```python
from build123d import *

# Parameters (mm, degrees)
BOSS_EXTRUDE1_DEPTH = 23
SKETCH2_R           = 18.51
CUT_EXTRUDE1_DEPTH  = 24
SKETCH3_R           = 13.985
CUT_EXTRUDE2_DEPTH  = 7
BOSS_EXTRUDE2_DEPTH = 23
CUT_EXTRUDE3_DEPTH  = 83.130091318
SKETCH10_R          = 3.5
CUT_EXTRUDE5_DEPTH  = 42
CUT_EXTRUDE8_DEPTH  = 83.130091318
CUT_EXTRUDE9_DEPTH  = 9
SKETCH15_R          = 3.5
CUT_EXTRUDE10_DEPTH = 82.477158286


with BuildPart() as part:
    # Sketch1 → Boss-Extrude1 (new body)
    with BuildSketch(Plane(origin=(0, 0, 0), x_dir=(1, 0, 0), z_dir=(0, 1, 0))):
        with BuildLine():
            Line((-100.336081003, -13.275177251), (-7.836081003, 21.091368721))
            ThreePointArc((-7.836081003, 21.091368721), (0, 22.5), (7.836081003, 21.091368721))
            Line((7.836081003, 21.091368721), (100.336081003, -13.275177251))
            ThreePointArc((100.336081003, -13.275177251), (113.745786388, -41.773742524), (85.524728129, -55.758029845))
            Line((85.524728129, -55.758029845), (56.196116933, -46.194642944))
            Line((56.196116933, -46.194642944), (-56.196116933, -46.194642944))
            Line((-56.196116933, -46.194642944), (-85.524728129, -55.758029845))
            ThreePointArc((-85.524728129, -55.758029845), (-113.745786388, -41.773742524), (-100.336081003, -13.275177251))
        make_face()
    extrude(amount=BOSS_EXTRUDE1_DEPTH)

    # Sketch2 → Cut-Extrude1 (cut, through all)
    with BuildSketch(Plane(origin=(0, 23, 0), x_dir=(1, 0, 0), z_dir=(0, 1, 0))):
        with Locations((-92.5, -34.366545972)):
            Circle(SKETCH2_R)
        with Locations((92.5, -34.366545972)):
            Circle(SKETCH2_R)
    extrude(amount=-CUT_EXTRUDE1_DEPTH, mode=Mode.SUBTRACT)

    # Sketch3 → Cut-Extrude2 (cut)
    with BuildSketch(Plane(origin=(0, 23, 0), x_dir=(1, 0, 0), z_dir=(0, 1, 0))):
        Circle(SKETCH3_R)
    extrude(amount=-CUT_EXTRUDE2_DEPTH, mode=Mode.SUBTRACT)

    # Sketch4 → Boss-Extrude2 (add)
    with BuildSketch(Plane(origin=(0, 23, 0), x_dir=(1, 0, 0), z_dir=(0, 1, 0))):
        with BuildLine():
            Line((-113.444632068, -26.146303424), (-132.192515375, -33.11170876))
            Line((-132.192515375, -33.11170876), (-121.744407372, -61.233533721))
            Line((-121.744407372, -61.233533721), (-102.996524064, -54.268128385))
            ThreePointArc((-102.996524064, -54.268128385), (-113.591368721, -42.202626974), (-113.444632068, -26.146303424))
        make_face()
        with BuildLine():
            Line((113.444632068, -26.146303424), (132.192515375, -33.11170876))
            Line((132.192515375, -33.11170876), (121.744407372, -61.233533721))
            Line((121.744407372, -61.233533721), (102.996524064, -54.268128385))
            ThreePointArc((102.996524064, -54.268128385), (113.591368721, -42.202626974), (113.444632068, -26.146303424))
        make_face()
    extrude(amount=-BOSS_EXTRUDE2_DEPTH)

    # Sketch5 → Cut-Extrude3 (cut, through all)
    with BuildSketch(Plane(origin=(5.224054002, 0, 14.060912481), x_dir=(0.937394165, 0, -0.348270267), z_dir=(0.348270267, 0, 0.937394165))):
        with BuildLine():
            Line((-135.448316262, 0), (-135.448316262, 14))
            Line((-135.448316262, 14), (-126.448316262, 14))
            ThreePointArc((-126.448316262, 14), (-133.448316262, 7), (-126.448316262, 0))
            Line((-126.448316262, 0), (-135.448316262, 0))
        make_face()
    extrude(amount=-CUT_EXTRUDE3_DEPTH, mode=Mode.SUBTRACT)

    # Sketch10 → Cut-Extrude5 (cut)
    with BuildSketch(Plane(origin=(5.224054002, 0, 14.060912481), x_dir=(0.937394165, 0, -0.348270267), z_dir=(0.348270267, 0, 0.937394165))):
        with Locations((-126.448316262, 7)):
            Circle(SKETCH10_R)
    extrude(amount=-CUT_EXTRUDE5_DEPTH, mode=Mode.SUBTRACT)

    # Sketch13 → Cut-Extrude8 (cut, through all)
    with BuildSketch(Plane(origin=(-5.224054002, 0, 14.060912481), x_dir=(0.937394165, 0, 0.348270267), z_dir=(-0.348270267, 0, 0.937394165))):
        with BuildLine():
            Line((126.448316262, 14), (135.448316262, 14))
            Line((135.448316262, 14), (135.448316262, 0))
            Line((135.448316262, 0), (126.448316262, 0))
            ThreePointArc((126.448316262, 0), (133.448316262, 7), (126.448316262, 14))
        make_face()
    extrude(amount=-CUT_EXTRUDE8_DEPTH, mode=Mode.SUBTRACT)

    # Sketch14 → Cut-Extrude9 (cut)
    with BuildSketch(Plane(origin=(0, 23, 0), x_dir=(1, 0, 0), z_dir=(0, 1, 0))):
        Polygon((-56.196116933, -46.194642944), (-93.033770242, 18.702535116), (-179.483612129, -24.236128073), (-123.538544412, -84.420295749), align=None)
        Polygon((179.483612129, -24.236128073), (123.538544412, -84.420295749), (56.196116933, -46.194642944), (93.033770242, 18.702535116), align=None)
    extrude(amount=-CUT_EXTRUDE9_DEPTH, mode=Mode.SUBTRACT)

    # Sketch15 → Cut-Extrude10 (cut, through all)
    with BuildSketch(Plane(origin=(-5.224054002, 0, 14.060912481), x_dir=(0.937394165, 0, 0.348270267), z_dir=(-0.348270267, 0, 0.937394165))):
        with Locations((126.448316262, 7)):
            Circle(SKETCH15_R)
    extrude(amount=-CUT_EXTRUDE10_DEPTH, mode=Mode.SUBTRACT)


solid = part.part
```
Read the model definition and answer for the solid it produces. Units are mm, in the model's axes. A direction names the side the tool comes from. Coordinates: 2 decimals unless noted, no trailing zeros. Loops run counter-clockwise (first coordinate to the right, second up) from the corner with the lowest first, then second, coordinate; pieces in that order, holes last. Notation, with made-up numbers: (-28.75, 4.5) - (-6.75, 4.5) arc R15 cw to (-6.75, 22.5) - close; hole circle Ø5 at (0, 40.25). An arc over 180 degrees is marked (long way). Answer in a Markdown table with one row per item.
1. Straight lines are drawn through the part: line 1 (X direction, y = 3.25, z = 26); line 2 (X direction, y = 6.5, z = 33); line 3 (Y direction, x = -74, z = 44). For each, find the intervals that lie inside material, in ascending order.
Conclusion:
| item | result |
|---|---|
| line 1 | x = -113.39 to -109.01, -75.99 to 75.99, 109.01 to 113.39 |
| line 2 | x = -130.08 to -126.33, -118.94 to -110.96, -74.04 to 74.04, 110.96 to 118.94, 126.33 to 130.08 |
| line 3 | y = 0 to 14 |
2. Find section C-C, the plane x = 0. Write down the section's boundary in (y, z) (3 decimals), then the cut area to 3 significant figures.
Conclusion:
| item | result |
|---|---|
| outline | (0, -22.5) - (23, -22.5) - (23, -13.985) - (16, -13.985) - (16, 13.985) - (23, 13.985) - (23, 46.195) - (0, 46.195) - close |
| area | 1,380 mm² |
3. Given pin 1 (6 mm diameter, centred on x = -99, y = 3.5, fed in from -Z); pin 2 (4 mm diameter, centred on y = 10.5, z = 15.5, fed in from -X); pin 3 (8 mm diameter, centred on x = -98.5, y = 11.5, fed in from +Z), each flat-ended and moving along its own axis, determine where each tip first touches the part or whether it passes through.
Conclusion:
| item | result |
|---|---|
| pin 1 | stops at z = 11.66 |
| pin 2 | stops at x = -107.39 |
| pin 3 | stops at z = 56.78 |
4. Find section D-D, the plane x = -106. Write down the section's boundary in (y, z).
Conclusion:
| item | result |
|---|---|
| outline | (0, 16.37) - (14, 16.37) - (14, 21.7) - (0, 21.7) - close; (0, 47.03) - (14, 47.03) - (14, 55.38) - (0, 55.38) - close |
5. Which of the six approach directions +Z, -Z, +X, -X, +Y, -Y give full straight-line access (tool end or side, diameter ignored) to faces 4 (the face through (71.066, 6.902, 51.043)), 5 (the face through (13.34, 19.55, -4.2)), 6 (the face through (-75, 14, 43))?
Conclusion:
| item | result |
|---|---|
| face 4 | +Z, +Y, -Y |
| face 5 | +Y |
| face 6 | +Z, -X, +Y |
6. Find section A-A, the plane x = 92.5. Write down the section's boundary in (y, z), then the cut area to 3 significant figures.
Conclusion:
| item | result |
|---|---|
| outline | (0, 10.36) - (14, 10.36) - (14, 15.86) - (0, 15.86) - close; (0, 52.88) - (14, 52.88) - (14, 56.87) - (0, 56.87) - close |
| area | 133 mm² |
7. Determine the mould class of faces 1 (the face through (2, 0, 26)), 2 (the face through (-74.845, 7.098, 28.807)), 3 (the face through (67.59, 18.56, 26.12)) for opening direction X: +X half, -X half, draft (parallel to the pull), parting line (faces both ways), or undercut.
Conclusion:
| item | result |
|---|---|
| face 1 | draft |
| face 2 | undercut |
| face 3 | +X half |
8. Find section B-B, the plane z = 10. Write down the section's boundary in (x, y), then the cut area to 3 significant figures.
Conclusion:
| item | result |
|---|---|
| outline | (-91.52, 0) - (91.52, 0) - (91.52, 14) - (76.74, 14) - (76.74, 23) - (9.78, 23) - (9.78, 16) - (-9.78, 16) - (-9.78, 23) - (-76.74, 23) - (-76.74, 14) - (-91.52, 14) - close |
| area | 3,810 mm² |
